Design review of the part built by this model. Coordinates are the model's own, in mm. A direction names the side the tool comes from. Give positions to 0.01 mm unless a question says otherwise; leave off trailing zeros. Write each loop counter-clockwise with the first axis right and the second up, starting at its lowest first coordinate (ties: lowest second). Pieces come first, ordered by that corner, then holes. Notation, with made-up numbers: M 26.5,82 L 33.5,82 A7 cw 33.5,92 Z; hole C 28.5,-15 d2. An arc over 180 degrees is marked long. Use one line per item in the form item = value. Start each with the question number.
from build123d import *

# Parameters (mm, degrees)
F0_R        = 6.5
F0_R_2      = 11.05
F1_DEPTH    = 9.2
F2_R        = 7.5
F2_R_2      = 4.4268339864
F2_R_3      = 11.05
F3_DEPTH    = 2
F4_R        = 2
F6_DEPTH    = 25
F7_SIZE     = 1
F8_C1_SIZE  = 1
F8_C2_SIZE  = 1
F8_C3_SIZE  = 1
F8_C4_SIZE  = 1
F8_C5_SIZE  = 1
F8_C6_SIZE  = 1
F8_C7_SIZE  = 1
F8_C8_SIZE  = 1
F8_C9_SIZE  = 1
F8_C10_SIZE = 1
F8_C11_SIZE = 1
F8_C12_SIZE = 1
F8_C13_SIZE = 1
F8_C14_SIZE = 1
F8_C15_SIZE = 1
F8_C16_SIZE = 1


with BuildPart() as f1:
    # F0 (on Front) → F1 (new body)
    with BuildSketch(Plane.XZ):
        with BuildLine():
            Line((-10.8594483096, 14.3268800737), (-2.4829795671, 13.8288579597))
            ThreePointArc((-2.4829795671, 13.8288579597), (-12.1676569232, 7.025), (-13.217632082, -4.7641055977))
            Line((-13.217632082, -4.7641055977), (-17.8371662556, 2.2411180703))
            ThreePointArc((-17.8371662556, 2.2411180703), (-34.6870755728, -20.0265924193), (-6.977717946, -16.5679981441))
            Line((-6.977717946, -16.5679981441), (-10.7346525149, -9.064752362))
            ThreePointArc((-10.7346525149, -9.064752362), (0, -14.05), (10.7346525149, -9.064752362))
            Line((10.7346525149, -9.064752362), (6.977717946, -16.5679981441))
            ThreePointArc((6.977717946, -16.5679981441), (34.6870755728, -20.0265924193), (17.8371662556, 2.2411180703))
            Line((17.8371662556, 2.2411180703), (13.217632082, -4.7641055977))
            ThreePointArc((13.217632082, -4.7641055977), (12.1676569232, 7.025), (2.4829795671, 13.8288579597))
            Line((2.4829795671, 13.8288579597), (10.8594483096, 14.3268800737))
            ThreePointArc((10.8594483096, 14.3268800737), (0, 40.0531848387), (-10.8594483096, 14.3268800737))
        make_face()
        with Locations((-21.5623582929, -12.4490333648)):
            Circle(F0_R, mode=Mode.SUBTRACT)
        with Locations((21.5623582929, -12.4490333648)):
            Circle(F0_R, mode=Mode.SUBTRACT)
        Circle(F0_R_2, mode=Mode.SUBTRACT)
        with Locations((0, 24.8980667296)):
            Circle(F0_R, mode=Mode.SUBTRACT)
    extrude(amount=F1_DEPTH)

    # F2 (on face) → F3 (join)
    with BuildSketch(Plane.XZ.offset(9.2)):
        with Locations((0, 24.8980667296)):
            Circle(F2_R)
        with Locations((0, 24.8980667296)):
            Circle(F2_R_2, mode=Mode.SUBTRACT)
        with Locations((-21.5623582929, -12.4490333648)):
            Circle(F2_R)
        with Locations((-21.5623582929, -12.4490333648)):
            Circle(F2_R_2, mode=Mode.SUBTRACT)
        with Locations((21.5623582929, -12.4490333648)):
            Circle(F2_R)
        with Locations((21.5623582929, -12.4490333648)):
            Circle(F2_R_2, mode=Mode.SUBTRACT)
        Circle(F2_R_3)
        Circle(F2_R, mode=Mode.SUBTRACT)
    extrude(amount=-F3_DEPTH)

    # F4
    f4_edges = [f1.edges().sort_by_distance(p)[0] for p in [
        (2.48298, -4.6, 13.828858),
        (-2.48298, -4.6, 13.828858),
        (-13.217632, -4.6, -4.764106),
        (-10.734653, -4.6, -9.064752),
        (10.734653, -4.6, -9.064752),
        (13.217632, -4.6, -4.764106),
    ]]
    fillet(f4_edges, radius=F4_R)

    # F5 (on face) → F6 (cut)
    with BuildSketch(Plane.XZ.offset(9.2)):
        with BuildLine():
            Line((0, 18.9108662307), (1.7659365324, 21.1738422452))
            ThreePointArc((1.7659365324, 21.1738422452), (0, 24.9152206672), (-1.7659365324, 21.1738422452))
            Line((-1.7659365324, 21.1738422452), (0, 18.9108662307))
        make_face()
        with BuildLine():
            Line((-16.3772905634, -9.4554331154), (-19.2200535463, -9.057575224))
            ThreePointArc((-19.2200535463, -9.057575224), (-21.5772140387, -12.4576103336), (-17.4541170138, -12.1162670212))
            Line((-17.4541170138, -12.1162670212), (-16.3772905634, -9.4554331154))
        make_face()
        with BuildLine():
            Line((16.3772905634, -9.4554331154), (17.4541170138, -12.1162670212))
            ThreePointArc((17.4541170138, -12.1162670212), (21.5772140387, -12.4576103336), (19.2200535463, -9.057575224))
            Line((19.2200535463, -9.057575224), (16.3772905634, -9.4554331154))
        make_face()
    extrude(amount=-F6_DEPTH, mode=Mode.SUBTRACT)

    # F7
    f7_edges = [f1.edges().sort_by_distance(p)[0] for p in [
        (10.530932, 0, 14.307348),
        (8.422362, 0, 12.919623),
        (0, 0, 40.053185),
        (12.167657, 0, 7.025),
        (-10.530932, 0, 14.307348),
        (15.399903, 0, 0.834168),
        (-8.422362, 0, 12.919623),
        (17.655993, 0, 1.96638),
        (-12.167657, 0, 7.025),
        (34.687076, 0, -20.026592),
        (-15.399903, 0, 0.834168),
        (7.125061, 0, -16.273728),
        (-17.655993, 0, 1.96638),
        (6.977541, 0, -13.753791),
        (-34.687076, 0, -20.026592),
        (0, 0, -14.05),
        (-7.125061, 0, -16.273728),
        (-6.977541, 0, -13.753791),
        (-28.062358, 0, -12.449033),
        (15.062358, 0, -12.449033),
        (-11.05, 0, 0),
        (-6.5, 0, 24.898067),
    ]]
    chamfer(f7_edges, length=F7_SIZE)

    # F8: chamfer of 1 on 28 edges, made by hand

    # F8_c1
    f8_c1_edges = [f1.edges().sort_by_distance(p)[0] for p in [
        (10.5309316289, -9.2, 14.3073481472),
        (8.4223621743, -9.2, 12.9196228952),
        (17.6559927707, -9.2, 1.9663802425),
        (15.3999027217, -9.2, 0.8341681552),
        (12.1676569232, -9.2, 7.025),
    ]]
    chamfer(f8_c1_edges, length=F8_C1_SIZE)

    # F8_c2
    f8_c2_edges = [f1.edges().sort_by_distance(p)[0] for p in [
        (-10.5309316289, -9.2, 14.3073481472),
        (-8.4223621743, -9.2, 12.9196228952),
        (-12.1676569232, -9.2, 7.025),
        (-15.3999027217, -9.2, 0.8341681552),
        (-17.6559927707, -9.2, 1.9663802425),
    ]]
    chamfer(f8_c2_edges, length=F8_C2_SIZE)

    # F8_c3
    f8_c3_edges = [f1.edges().sort_by_distance(p)[0] for p in [
        (-7.1250611419, -9.2, -16.2737283897),
        (-6.9775405475, -9.2, -13.7537910504),
        (0, -9.2, -14.05),
        (6.9775405475, -9.2, -13.7537910504),
        (7.1250611419, -9.2, -16.2737283897),
    ]]
    chamfer(f8_c3_edges, length=F8_C3_SIZE)

    # F8_c4
    f8_c4_edges = [f1.edges().sort_by_distance(p)[0] for p in [
        (34.6870755728, -9.2, -20.0265924193),
    ]]
    chamfer(f8_c4_edges, length=F8_C4_SIZE)

    # F8_c5
    f8_c5_edges = [f1.edges().sort_by_distance(p)[0] for p in [
        (-25.3961089835, -9.2, -14.662450358),
    ]]
    chamfer(f8_c5_edges, length=F8_C5_SIZE)

    # F8_c6
    f8_c6_edges = [f1.edges().sort_by_distance(p)[0] for p in [
        (-16.7411021229, -9.2, -9.4045159968),
    ]]
    chamfer(f8_c6_edges, length=F8_C6_SIZE)

    # F8_c7
    f8_c7_edges = [f1.edges().sort_by_distance(p)[0] for p in [
        (-16.515100825, -9.2, -9.7959617274),
    ]]
    chamfer(f8_c7_edges, length=F8_C7_SIZE)

    # F8_c8
    f8_c8_edges = [f1.edges().sort_by_distance(p)[0] for p in [
        (25.3961089835, -9.2, -14.662450358),
    ]]
    chamfer(f8_c8_edges, length=F8_C8_SIZE)

    # F8_c9
    f8_c9_edges = [f1.edges().sort_by_distance(p)[0] for p in [
        (16.515100825, -9.2, -9.7959617274),
    ]]
    chamfer(f8_c9_edges, length=F8_C9_SIZE)

    # F8_c10
    f8_c10_edges = [f1.edges().sort_by_distance(p)[0] for p in [
        (16.7411021229, -9.2, -9.4045159968),
    ]]
    chamfer(f8_c10_edges, length=F8_C10_SIZE)

    # F8_c11
    f8_c11_edges = [f1.edges().sort_by_distance(p)[0] for p in [
        (-7.5, -9.2, 0),
    ]]
    chamfer(f8_c11_edges, length=F8_C11_SIZE)

    # F8_c12
    f8_c12_edges = [f1.edges().sort_by_distance(p)[0] for p in [
        (0, -9.2, 29.324900716),
    ]]
    chamfer(f8_c12_edges, length=F8_C12_SIZE)

    # F8_c13
    f8_c13_edges = [f1.edges().sort_by_distance(p)[0] for p in [
        (0.226001298, -9.2, 19.2004777242),
    ]]
    chamfer(f8_c13_edges, length=F8_C13_SIZE)

    # F8_c14
    f8_c14_edges = [f1.edges().sort_by_distance(p)[0] for p in [
        (-0.226001298, -9.2, 19.2004777242),
    ]]
    chamfer(f8_c14_edges, length=F8_C14_SIZE)

    # F8_c15
    f8_c15_edges = [f1.edges().sort_by_distance(p)[0] for p in [
        (0, -9.2, 40.0531848387),
    ]]
    chamfer(f8_c15_edges, length=F8_C15_SIZE)

    # F8_c16
    f8_c16_edges = [f1.edges().sort_by_distance(p)[0] for p in [
        (-34.6870755728, -9.2, -20.0265924193),
    ]]
    chamfer(f8_c16_edges, length=F8_C16_SIZE)


solid = f1.part
1. For faces 1 (the cylindrical face through (-15.37, -4.65, 0.84)), 2 (the flat face through (-16.243, -8.693, -10.438)), 3 (the cylindrical face through (-2.395, -4.057, -10.787)), list the 3-axis set-ups (+Z, -Z, +X, -X, +Y, -Y) from which the entire face can be reached by the end or side of a thin tool; tool diameter is ignored.
2. Clearance check with flat-ended pins moving along their axes: pin 1 Ø10 at (x, z) = (0, 24.9) entering from +Y; pin 2 Ø4 at (y, z) = (-3.5, 5.5) entering from -X; pin 3 Ø2 at (y, z) = (-8, 17.5) entering from +X; pin 4 Ø4 at (x, z) = (-1.5, 26) entering from +Y. State where each tip first meets the part, or that it passes through.
3. We need section A-A (y = -4.5). State the section outline as (x, z) points (3 decimals).
4. Draft analysis for pull direction X (two halves, no side actions). For faces 4 (the conical face through (0.47, -0.174, 39.219)), 5 (the cylindrical face through (-7, -4.65, -13.78)), 6 (the cylindrical face through (8.433, -4.65, 12.951)), state which applies: pulls with the +X half, pulls with the -X half, needs draft (parallel to the pull), parting line crosses it, or undercut.
5. To check wall thickness, follow L1, parallel to X at y = -7.5, z = -3.5; L2, parallel to Z at x = 9, y = -8; L3, parallel to Z at x = 23, y = -3. State the ranges of each line that lie inside material, in increasing order.
6. We need section B-B (x = 3). Give the number of separate pieces and of enclosed holes in the cut face, and give its area (3 significant figures).
Answer block:
q1.face_1 = +Y, -Y
q1.face_2 = -Y
q1.face_3 = +Y
q2.pin_1 = -7.2
q2.pin_2 = -13.61
q2.pin_3 = 13.74
q2.pin_4 = through
q3.outline = M -17.837,2.241 A15.155 ccw long -6.978,-16.568 L -7.272,-15.979 A2 cw -4.801,-13.204 A14.05 ccw 4.801,-13.204 A2 cw 7.272,-15.979 L 6.978,-16.568 A15.155 ccw long 17.837,2.241 L 17.475,1.692 A2 cw 13.836,2.445 A14.05 ccw 9.035,10.76 A2 cw 10.202,14.288 L 10.859,14.327 A15.155 ccw long -10.859,14.327 L -10.202,14.288 A2 cw -9.035,10.76 A14.05 ccw -13.836,2.445 A2 cw -17.475,1.692 Z; hole C -21.562,-12.449 d13; hole C 0,0 d22.1; hole C 0,24.898 d13; hole C 21.562,-12.449 d13
q4.face_4 = parting line crosses it
q4.face_5 = undercut
q4.face_6 = pulls with the +X half
q5.L1 = -33.79 to -6.63, 6.63 to 33.79
q5.L2 = -20.93 to 10.79, 13.79 to 37.09
q5.L3 = -27.54 to -18.79, -6.11 to 2.64
q6.separate_pieces = 3
q6.enclosed_holes = 0
q6.area = 209 mm^2
